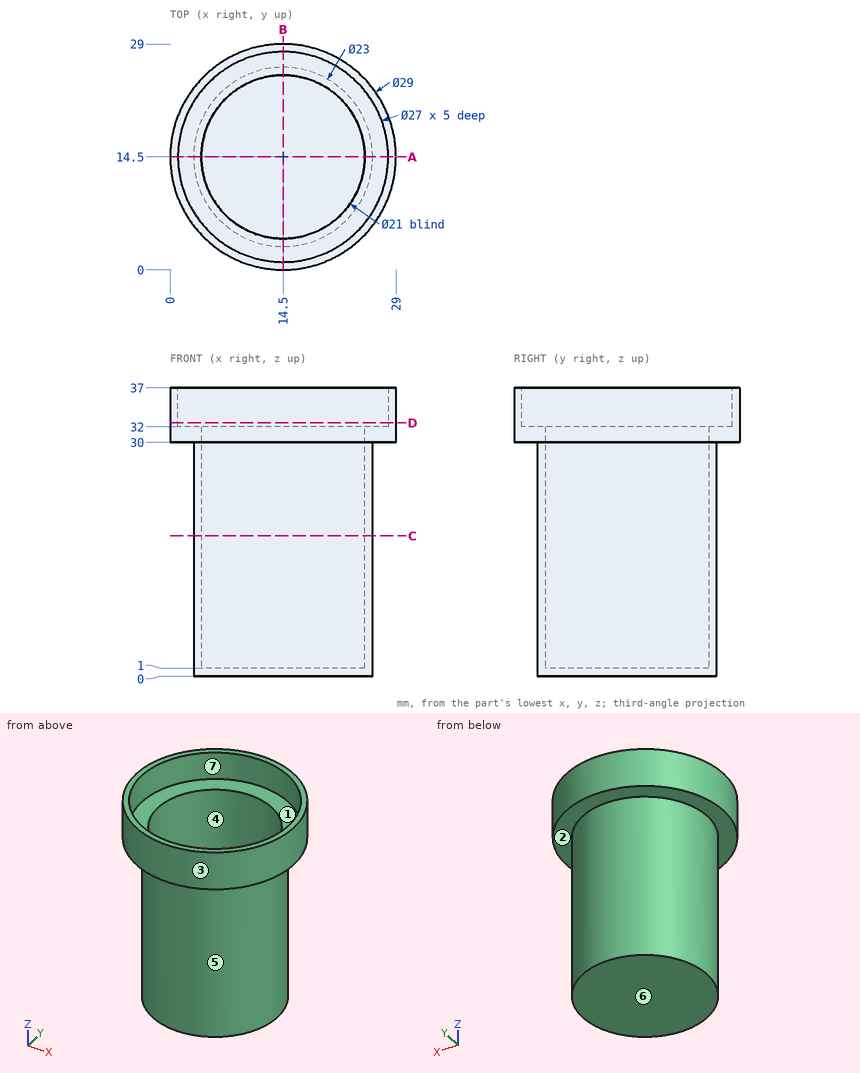
Study the drawing (mm; zero at the part's minimum x, y, z) and answer. A direction names the side the tool comes from. Give positions to 0.01 mm unless a question says otherwise; leave off trailing zeros. Order: outer loops, then holes, each group sorted by start corner. A loop starts at its lowest first (then second) coordinate and runs counter-clockwise, first axis right, second up. Notation, with made-up numbers: M -19.75,-29 L 11.25,-29 A13 ccw 11.25,-8 Z; hole C 45.25,-1 d9. An arc over 180 degrees is marked long. Put each result on its own line as item: value. Start each with the question number.
Item 1: Find the intervals of material crossed by line 1 along Y through (x, z) = (14.5, 36.05); line 2 along Z through (x, y) = (15.75, 11); line 3 along Y through (x, z) = (14.5, 23.5), in increasing order.
Item 2: The part is cut by section D-D, the plane z = 32.5. Determine the outline of the cut face in (x, y), and give its area (3 significant figures).
Item 3: The part is cut by section C-C, the plane z = 18. Determine the outline of the cut face in (x, y), and give its area (3 significant figures).
Item 4: Flat-ended cylindrical pins translate along their axes: P1, Ø2, axis at y = 12.5, z = 17.5, coming from the -X side; P2, Ø5, axis at x = 14.5, z = 5, coming from the -Y side; P3, Ø6, axis at x = 13, y = 16, coming from the -Z side; P4, Ø2, axis at y = 13, z = 17, coming from the +X side. Find the tip coordinate at first contact, or state that the pin passes through.
Item 5: For a pull along Y with two mould halves and no side action, classify the marked faces 4, 5, 6 and 7 as +Y half, -Y half, draft (parallel to the pull), parting line (faces both ways), or undercut.
Item 6: Which of the six approach directions +Z, -Z, +X, -X, +Y, -Y give full straight-line access (tool end or side, diameter ignored) to the marked faces 1, 2 and 3?
Item 7: The part is cut by section A-A, the plane y = 14.5. Determine the outline of the cut face in (x, z).
Answer key:
1. line 1: y = 0 to 1, 28 to 29
1. line 2: z = 0 to 1
1. line 3: y = 3 to 4, 25 to 26
2. outline: C 14.5,14.5 d29; hole C 14.5,14.5 d27
2. area: 88.0 mm²
3. outline: C 14.5,14.5 d23; hole C 14.5,14.5 d21
3. area: 69.1 mm²
4. P1: stops at x = 3.04
4. P2: stops at y = 3
4. P3: stops at z = 0
4. P4: stops at x = 25.99
5. face 4: undercut
5. face 5: parting line
5. face 6: draft
5. face 7: undercut
6. face 1: +Z
6. face 2: -Z
6. face 3: +Z, -Z
7. outline: M 0,30 L 3,30 L 3,0 L 26,0 L 26,30 L 29,30 L 29,37 L 28,37 L 28,32 L 25,32 L 25,1 L 4,1 L 4,32 L 1,32 L 1,37 L 0,37 Z
